Geometry: see drawing. Coordinates: mm, zero at the bounding-box minimum. Coordinates: 2 decimals unless noted, no trailing zeros. Order: outer loops, then holes, each group sorted by start corner. A loop starts at its lowest first (then second) coordinate and runs counter-clockwise, first axis right, second up. Notation, with made-up numbers: M 75,-5.75 L 101,-5.75 A15 cw 101,21.25 Z; hole C 76,58 d3. An arc over 180 degrees is marked long. Answer in a Markdown table with one row per item.
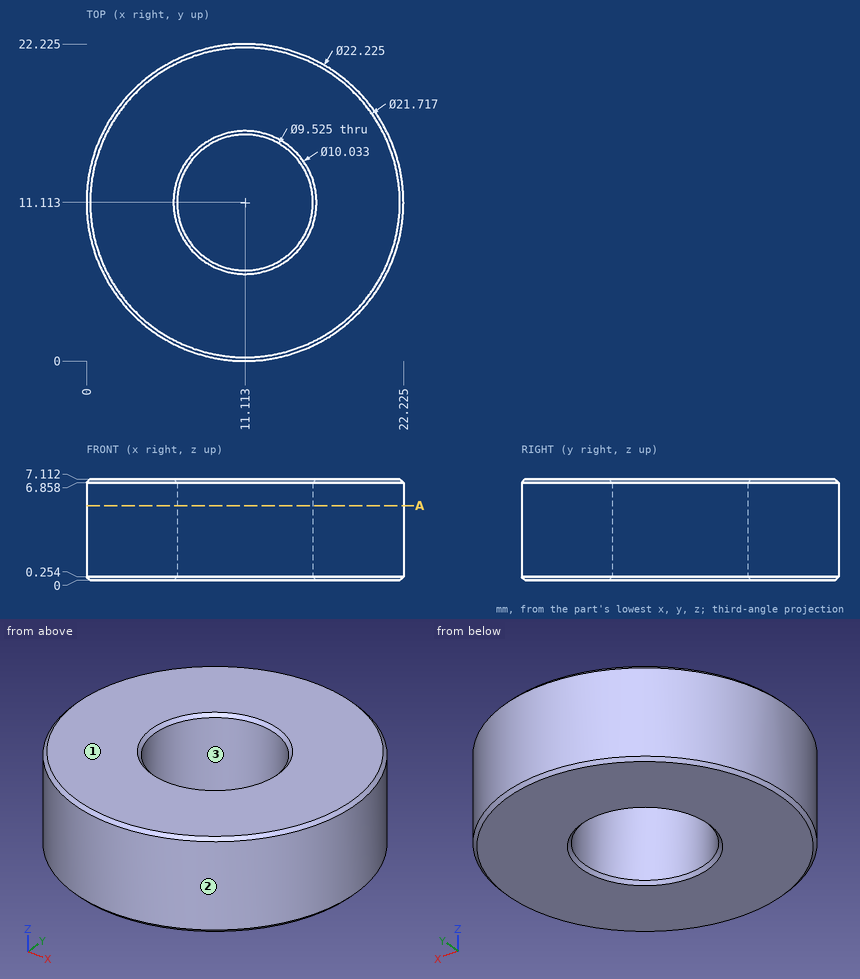
1) Material intervals for probe 1 along X at (y, z) = (14.5, 1.5) (1 decimal); probe 2 along X at (y, z) = (6.75, 4) (1 decimal); probe 3 along Y at (x, z) = (9, 1) (1 decimal), sorted ascending.
Resolved:
| item | result |
|---|---|
| probe 1 | x = 0.5 to 7.8, 14.5 to 21.7 |
| probe 2 | x = 0.9 to 9.2, 13 to 21.3 |
| probe 3 | y = 0.2 to 6.8, 15.4 to 22 |
2) Mould query, pull axis X, two halves, no side actions, for the marked faces 1, 2 and 3. Classes: +X half, -X half, draft (parallel to the pull), parting line (faces both ways), or undercut.
Resolved:
| item | result |
|---|---|
| face 1 | draft |
| face 2 | parting line |
| face 3 | undercut |
3) Cut plane A-A, the plane z = 5.25. Output: boundary loops of the cut face in (x, y) (1 decimal), and give its area (3 significant figures).
Resolved:
| item | result |
|---|---|
| outline | C 11.1,11.1 d22.2; hole C 11.1,11.1 d9.5 |
| area | 317 mm2 |
4) Contact query for flat-ended pins moving along their axis: pin 1 (2 mm diameter, centred on y = 19, z = 3.5, fed in from -X); pin 2 (2 mm diameter, centred on y = 17, z = 2.5, fed in from +X). Output: stop coordinate, or through.
Resolved:
| item | result |
|---|---|
| pin 1 | stops at x = 2.39 |
| pin 2 | stops at x = 21.09 |
